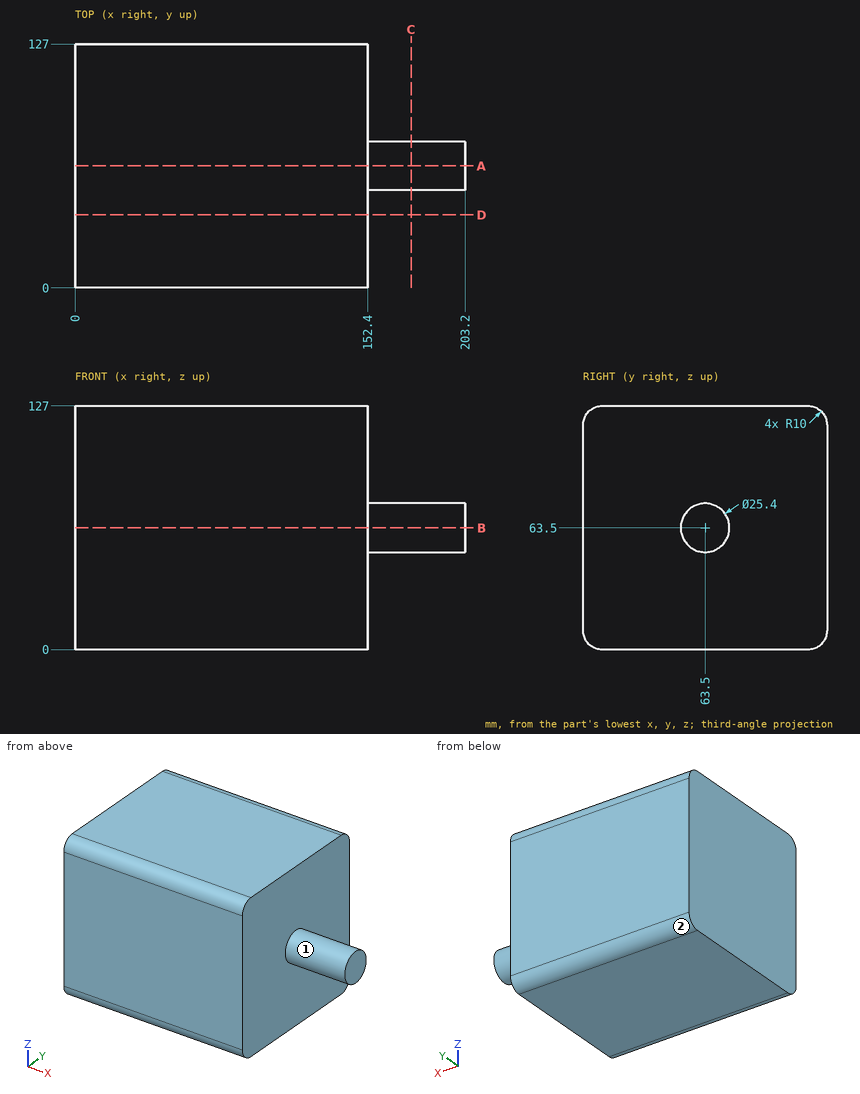
Answer from the drawing. Dimensions are ordinates in mm from the lowest x, y and z of the part. A direction names the side the tool comes from. Coordinates: 2 decimals unless noted, no trailing zeros. Write each loop counter-clockwise with the first axis right and the second up, starting at its lowest first coordinate (ties: lowest second). Pieces come first, ordered by that corner, then holes. Notation, with made-up numbers: (65.5, 36.5) - (117.5, 36.5) arc R21 cw to (117.5, 64.5) - close; hole circle Ø4 at (-39, 85). An arc over 180 degrees is marked (long way). Return JSON: item names as keys, results as strings.
1. Consider line 1 along X through (y, z) = (74, 17); line 2 along Z through (x, y) = (77.5, 9.5); line 3 along Z through (x, y) = (155, 67). Determine where each line is inside the solid, lowest interval first.
Final values:
{"line 1": "0 to 152.4", "line 2": "0.01 to 126.99", "line 3": "51.29 to 75.71"}
2. The part is cut by section D-D on y = 38. Determine the outline of the cut face in (x, z), then the cut area to 3 significant figures.
Final values:
{"outline": "(0, 0) - (152.4, 0) - (152.4, 127) - (0, 127) - close", "area": "19,400 mm^2"}
3. The part is cut by section A-A on y = 63.5. Determine the outline of the cut face in (x, z), then the cut area to 3 significant figures.
Final values:
{"outline": "(0, 0) - (152.4, 0) - (152.4, 50.8) - (203.2, 50.8) - (203.2, 76.2) - (152.4, 76.2) - (152.4, 127) - (0, 127) - close", "area": "20,600 mm^2"}
4. The part is cut by section C-C on x = 175. Determine the outline of the cut face in (y, z), then the cut area to 3 significant figures.
Final values:
{"outline": "circle Ø25.4 at (63.5, 63.5)", "area": "507 mm^2"}
5. Which of the six approach directions +Z, -Z, +X, -X, +Y, -Y give full straight-line access (tool end or side, diameter ignored) to the marked faces 1 and 2?
Final values:
{"face 1": "+X", "face 2": "-Z, +X, -X, +Y"}
6. This flat-tipped pin is pushed along its axis until it touches: pin 1 Ø2 at (y, z) = (94.5, 57) entering from +X. Where does it stop, or does it pass through?
Final values:
{"pin 1": "x = 152.4"}
